from build123d import *

# Parameters (mm, degrees)
F0_W      = 304.8
F0_H      = 127
F1_DEPTH  = 38.1
F2_W      = 31.75
F2_H      = 127
F3_DEPTH  = 63.5
F5_DEPTH  = 127.001
F7_DEPTH  = 273.05
F9_DEPTH  = 38.1
F10_R     = 12.7
F11_DEPTH = 38.1


with BuildPart() as f1:
    # F0 (on Top) → F1 (new body)
    with BuildSketch(Plane.XY):
        with Locations((152.4, 63.5)):
            Rectangle(F0_W, F0_H)
    extrude(amount=F1_DEPTH)

    # F2 (on face) → F3 (join)
    with BuildSketch(Plane.XY.offset(38.1)):
        with Locations((15.875, 63.5)):
            Rectangle(F2_W, F2_H)
    extrude(amount=F3_DEPTH)

    # F4 (on face) → F5 (cut, through all)
    with BuildSketch(Plane.XZ):
        Polygon((19.05, 101.6), (0, 101.6), (0, 82.55), align=None)
    extrude(amount=-F5_DEPTH, mode=Mode.SUBTRACT)

    # F6 (on face) → F7 (cut)
    with BuildSketch(Plane.YZ.offset(304.8)):
        Polygon((50.8, 16.51), (50.8, 0), (76.2, 0), (76.2, 16.51), (95.25, 16.51), (95.25, 29.21), (76.2, 29.21), (76.2, 38.1), (50.8, 38.1), (50.8, 29.21), (31.75, 29.21), (31.75, 16.51), align=None)
    extrude(amount=-F7_DEPTH, mode=Mode.SUBTRACT)

    # F8 (on face) → F9 (join)
    with BuildSketch(Plane.YZ.offset(304.8)):
        with BuildLine():
            Line((0, 50.8), (0, 38.1))
            Line((0, 38.1), (127, 38.1))
            Line((127, 38.1), (127, 50.8))
            Line((127, 50.8), (111.125, 50.8))
            Line((111.125, 50.8), (84.360147, 90.419272))
            ThreePointArc((84.360147, 90.419272), (63.22985, 101.600555), (42.17301, 90.281542))
            Line((42.17301, 90.281542), (15.875, 50.8))
            Line((15.875, 50.8), (0, 50.8))
        make_face()
    extrude(amount=-F9_DEPTH)

    # F10 (on face) → F11 (cut)
    with BuildSketch(Plane.YZ.offset(304.8)):
        with Locations((63.312774, 76.20069)):
            Circle(F10_R)
    extrude(amount=-F11_DEPTH, mode=Mode.SUBTRACT)


solid = f1.part
Geometry: final body of the model. Coordinates: model frame, mm. A direction names the side the tool comes from. Give positions to 0.01 mm unless a question says otherwise; leave off trailing zeros. Loops run counter-clockwise (first coordinate to the right, second up) from the corner with the lowest first, then second, coordinate; pieces in that order, holes last. Notation, with made-up numbers: M 85.25,-22.5 L 104.25,-22.5 A24 cw 104.25,10.5 Z; hole C -21,40.25 d9. An arc over 180 degrees is marked long. Put each result on its own line as item: value. Start each with the question number.
1) Contact query for flat-ended pins moving along their axis: pin 1 (5 mm diameter, centred on x = 283.5, y = 120, fed in from +Z); pin 2 (8 mm diameter, centred on y = 68, z = 19, fed in from +X); pin 3 (5.5 mm diameter, centred on x = 202.5, y = 84.5, fed in from +Z). Output: stop coordinate, or through.
2) Cut plane B-B (z = 46). Output: boundary loops of the cut face in (x, y).
3) Pull-direction query (Z, two-part tool) for faces 6 (the flat face through (286.02, 97.93, 70.33)), 7 (the flat face through (150, 50, 0)), 8 (the flat face through (170, 41, 16.51)), 9 (the flat face through (0, 63, 41)); classes: pulls with the +Z half, pulls with the -Z half, needs draft (parallel to the pull), parting line crosses it, or undercut.
4) Access query for faces 1 (the cylindrical face through (286, 63.6, 101.6)), 2 (the flat face through (286, 119, 50.8)), 3 (the flat face through (148, 26, 38.1)), 4 (the flat face through (170, 41, 29.21)), 5 (the flat face through (286.02, 29.21, 70.82)). Directions: +Z, -Z, +X, -X, +Y, -Y. A direction counts if a zero-diameter tool reaches every point of the face in a straight line with its end or side. Return the directions, or none.
5) Cut plane A-A (x = 135.5). Output: boundary loops of the cut face in (y, z).
6) Ray query, line 1 along Z through (x, y) = (243, 78); line 2 along Y through (x, z) = (106, 12); line 3 along X through (y, z) = (79, 54). Return the intervals inside material, ascending.
7) Cut plane C-C (z = 22). Output: boundary loops of the cut face in (x, y), then the cut area to 3 significant figures.
8) Cut plane D-D (y = 64.5). Output: boundary loops of the cut face in (x, z).
Verdict:
1. pin 1: z = 50.8
1. pin 2: x = 31.75
1. pin 3: z = 38.1
2. outline: M 0,0 L 31.75,0 L 31.75,127 L 0,127 Z; M 266.7,0 L 304.8,0 L 304.8,127 L 266.7,127 Z
3. face 6: pulls with the +Z half
3. face 7: pulls with the -Z half
3. face 8: undercut
3. face 9: needs draft
4. face 1: +Z, +X
4. face 2: +Z, +X, +Y
4. face 3: +Z, +Y, -Y
4. face 4: +X
4. face 5: +Z, +X, -Y
5. outline: M 0,0 L 50.8,0 L 50.8,16.51 L 31.75,16.51 L 31.75,29.21 L 50.8,29.21 L 50.8,38.1 L 0,38.1 Z; M 76.2,0 L 127,0 L 127,38.1 L 76.2,38.1 L 76.2,29.21 L 95.25,29.21 L 95.25,16.51 L 76.2,16.51 Z
6. line 1: 0 to 16.51, 29.21 to 38.1
6. line 2: 0 to 50.8, 76.2 to 127
6. line 3: 0 to 31.75, 266.7 to 304.8
7. outline: M 0,0 L 304.8,0 L 304.8,31.75 L 31.75,31.75 L 31.75,95.25 L 304.8,95.25 L 304.8,127 L 0,127 Z
7. area: 21,400 mm2
8. outline: M 0,0 L 31.75,0 L 31.75,101.6 L 19.05,101.6 L 0,82.55 Z; M 266.7,38.1 L 304.8,38.1 L 304.8,63.56 L 266.7,63.56 Z; M 266.7,88.85 L 304.8,88.85 L 304.8,101.57 L 266.7,101.57 Z
